Source: three-view drawing plus pictorial views. Frame: mm from the lowest corner of the part. A direction names the side the tool comes from. Give positions to 0.01 mm unless a question says otherwise; leave off trailing zeros. Loops run counter-clockwise (first coordinate to the right, second up) from the corner with the lowest first, then second, coordinate; pieces in that order, holes last.
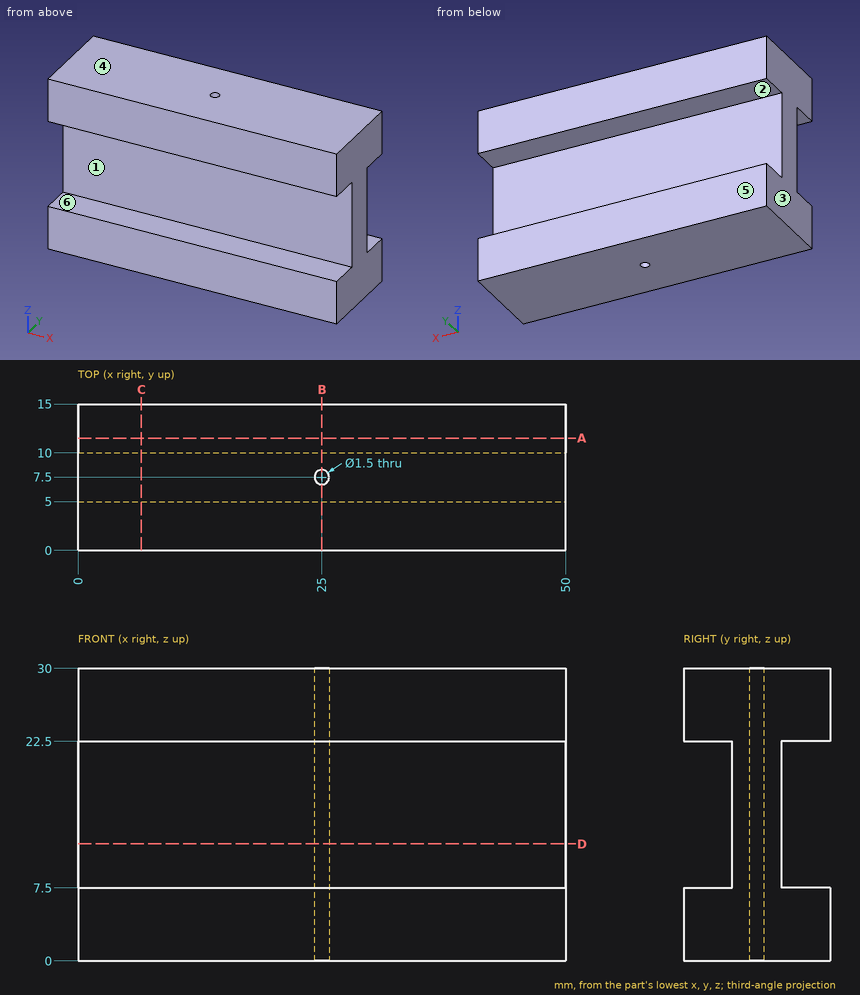
(1) Cut plane D-D (z = 12). Return the cut outline in (x, y).
Values follow:
outline: (0, 5) - (50, 5) - (50, 10) - (0, 10) - close; hole circle Ø1.5 at (25, 7.5)
(2) Pin query (flat end, axial travel): pin 1 Ø1.4 at (x, y) = (25, 7.5) entering from +Z; pin 2 Ø3 at (x, z) = (9, 10) entering from -Y; pin 3 Ø7.5 at (x, z) = (29.5, 13.5) entering from +Y. Return the tip coordinate at first contact, or that it passes through.
Values follow:
pin 1: passes through
pin 2: stops at y = 5
pin 3: stops at y = 10
(3) Cut plane B-B (x = 25). Return the cut outline in (y, z), and give its area (3 significant figures).
Values follow:
outline: (0, 0) - (6.75, 0) - (6.75, 30) - (0, 30) - (0, 22.5) - (5, 22.5) - (5, 7.5) - (0, 7.5) - close; (8.25, 0) - (15, 0) - (15, 7.5) - (10, 7.5) - (10, 22.5) - (15, 22.5) - (15, 30) - (8.25, 30) - close
area: 255 mm2
(4) Cut plane A-A (y = 11.5). Return the cut outline in (x, z), and give its area (3 significant figures).
Values follow:
outline: (0, 0) - (50, 0) - (50, 7.5) - (0, 7.5) - close; (0, 22.5) - (50, 22.5) - (50, 30) - (0, 30) - close
area: 750 mm2
(5) Mould query, pull axis Z, two halves, no side actions, for the marked faces 4, 5 and 6. Classes: +Z half, -Z half, draft (parallel to the pull), parting line (faces both ways), or undercut.
Values follow:
face 4: +Z half
face 5: draft
face 6: undercut
(6) Ray query, probe 1 along Z at (x, y) = (11, 11.5); probe 2 along Y at (x, z) = (25, 19.25); probe 3 along Y at (x, z) = (22.5, 9). Return the intervals inside material, ascending.
Values follow:
probe 1: z = 0 to 7.5, 22.5 to 30
probe 2: y = 5 to 6.75, 8.25 to 10
probe 3: y = 5 to 10
(7) Reachability of the marked faces 1, 2 and 3 from +Z, -Z, +X, -X, +Y, -Y: full face, straight path, thin tool, end or side. Return the list, or none.
Values follow:
face 1: +X, -X, -Y
face 2: +X, -X, +Y
face 3: +Z, -Z, -X, +Y, -Y
(8) Cut plane C-C (x = 6.5). Return the cut outline in (y, z).
Values follow:
outline: (0, 0) - (15, 0) - (15, 7.5) - (10, 7.5) - (10, 22.5) - (15, 22.5) - (15, 30) - (0, 30) - (0, 22.5) - (5, 22.5) - (5, 7.5) - (0, 7.5) - close
